CAD build for the part. Positions are in the model's coordinates, mm. A direction names the side the tool comes from. Round coordinates to 2 decimals unless told otherwise and drop trailing zeros. Loops run counter-clockwise (first coordinate to the right, second up) from the corner with the lowest first, then second, coordinate; pieces in that order, holes last. Notation, with made-up numbers: M -33,-7.5 L -11,-7.5 A8 ccw -11,5.5 Z; hole C -0.5,-2.75 d1. An arc over 180 degrees is marked long. Use a Markdown table: item, result. Add a question column.
(1) Band-saw the part on D-D, the plane y = 6.5. Write the cut outline in (x, z).
(2) Wall check: L1, parallel to Y at x = -15.5, z = 18.5; L2, parallel to Z at x = 10, y = -1.5; L3, parallel to Y at x = 0, z = 28. Give the ranges that are in metal, low to high.
(3) Which spindle directions (+Z, -Z, +X, -X, +Y, -Y) get a long thin tool onto all of the face, cutting with end or side? Do faces 4 (the face through (7.1, -12, 11)), 5 (the face through (0, -15, 16.5)), 6 (the face through (-0.508, 10.367, 19.74)). Say none if no direction does.
(4) Flat gauge pins, fed straight in: P1, Ø1, axis at x = -1, y = -14.5, coming from the +Z side; P2, Ø12, axis at y = -13, z = 10.5, coming from the -X side; P3, Ø2, axis at x = -0.5, y = -15, coming from the -Z side; P4, Ø10, axis at x = -11, y = -9.5, coming from the -Z side. Where does each tip first touch, or does it go through?
(5) Two-plate mould, pull along X, no slides. Class faces 1 (the face through (-1.56, 11.9, 9.37)), 2 (the face through (0, 7, 29)), 3 (the face through (13.4, 0.09, 18.61)): released by +X, released by -X, zero draft, split by the parting line, or undercut.
(6) Band-saw the part on C-C, the plane z = 25. Write the cut outline in (x, y).
(7) Band-saw the part on B-B, the plane x = 0. Write the cut outline in (y, z).
(8) Band-saw the part on A-A, the plane y = 0. Write the cut outline in (x, z), and give its area (3 significant figures).
from build123d import *

# Parameters (mm, degrees)
SKETCH1_R           = 12
BOSS_EXTRUDE1_DEPTH = 19
SKETCH2_R           = 3.9
BOSS_EXTRUDE2_DEPTH = 1.5
SKETCH3_R           = 2.1
BOSS_EXTRUDE3_DEPTH = 0.8
SKETCH4_R           = 2.5
BOSS_EXTRUDE4_DEPTH = 8.5
CUT_EXTRUDE2_DEPTH  = 6
SKETCH6_W           = 14.2
SKETCH6_H           = 16.3
BOSS_EXTRUDE5_DEPTH = 13.6
SKETCH7_W           = 7
SKETCH7_H           = 1
BOSS_EXTRUDE6_DEPTH = 2


with BuildPart() as part:
    # Sketch1 → Boss-Extrude1 (new body)
    with BuildSketch(Plane.XY):
        Circle(SKETCH1_R)
    extrude(amount=BOSS_EXTRUDE1_DEPTH)

    # Sketch2 → Boss-Extrude2 (add)
    with BuildSketch(Plane.XY.offset(19)):
        with Locations((0, 6.5)):
            Circle(SKETCH2_R)
    extrude(amount=BOSS_EXTRUDE2_DEPTH)

    # Sketch3 → Boss-Extrude3 (add)
    with BuildSketch(Plane.XY.offset(19)):
        with BuildLine():
            Line((-15.5, 3.5), (15.5, 3.5))
            ThreePointArc((15.5, 3.5), (19, 0), (15.5, -3.5))
            Line((15.5, -3.5), (-15.5, -3.5))
            ThreePointArc((-15.5, -3.5), (-19, 0), (-15.5, 3.5))
        make_face()
        with Locations((-15.5, 0)):
            Circle(SKETCH3_R, mode=Mode.SUBTRACT)
        with Locations((15.5, 0)):
            Circle(SKETCH3_R, mode=Mode.SUBTRACT)
    extrude(amount=-BOSS_EXTRUDE3_DEPTH)

    # Sketch4 → Boss-Extrude4 (add)
    with BuildSketch(Plane.XY.offset(20.5)):
        with Locations((0, 6.5)):
            Circle(SKETCH4_R)
    extrude(amount=BOSS_EXTRUDE4_DEPTH)

    # Sketch5 → Cut-Extrude2 (cut)
    with BuildSketch(Plane.XY.offset(29)):
        with BuildLine():
            Line((-2, 8), (2, 8))
            ThreePointArc((2, 8), (0, 9), (-2, 8))
        make_face()
        with BuildLine():
            Line((2, 5), (-2, 5))
            ThreePointArc((-2, 5), (0, 4), (2, 5))
        make_face()
    extrude(amount=-CUT_EXTRUDE2_DEPTH, mode=Mode.SUBTRACT)

    # Sketch6 → Boss-Extrude5 (add)
    with BuildSketch(Plane(origin=(0, 0, 0), x_dir=(1, 0, 0), z_dir=(0, 1, 0))):
        with Locations((0, -10.85)):
            Rectangle(SKETCH6_W, SKETCH6_H)
    extrude(amount=-BOSS_EXTRUDE5_DEPTH)

    # Sketch7 → Boss-Extrude6 (add)
    with BuildSketch(Plane.XZ.offset(13.6)):
        with Locations((-0.219512042, 17)):
            Rectangle(SKETCH7_W, SKETCH7_H)
    extrude(amount=BOSS_EXTRUDE6_DEPTH)


solid = part.part
Return value:
| question | item | result |
|---|---|---|
| 1 | outline | M -10.09,0 L 10.09,0 L 10.09,19 L 3.9,19 L 3.9,20.5 L 2.5,20.5 L 2.5,29 L -2.5,29 L -2.5,20.5 L -3.9,20.5 L -3.9,19 L -10.09,19 Z |
| 2 | L1 | -3.5 to -2.1, 2.1 to 3.5 |
| 2 | L2 | 0 to 19 |
| 2 | L3 | 5 to 8 |
| 3 | face 4 | +Z, -Z, +X, -Y |
| 3 | face 5 | -Z, +X, -X, -Y |
| 3 | face 6 | +Z |
| 4 | P1 | z = 17.5 |
| 4 | P2 | x = -9.75 |
| 4 | P3 | z = 16.5 |
| 4 | P4 | z = 0 |
| 5 | face 1 | split by the parting line |
| 5 | face 2 | zero draft |
| 5 | face 3 | undercut |
| 6 | outline | M -2,5 L 2,5 A2.5 ccw 2,8 L -2,8 A2.5 ccw Z |
| 7 | outline | M -15.6,16.5 L -13.6,16.5 L -13.6,2.7 L -12,2.7 L -12,0 L 12,0 L 12,19 L 10.4,19 L 10.4,20.5 L 9,20.5 L 9,23 L 8,23 L 8,29 L 5,29 L 5,23 L 4,23 L 4,20.5 L 2.6,20.5 L 2.6,19 L -13.6,19 L -13.6,17.5 L -15.6,17.5 Z |
| 8 | outline | M -19,18.2 L -17.6,18.2 L -17.6,19 L -19,19 Z; M -13.4,18.2 L -12,18.2 L -12,0 L 12,0 L 12,18.2 L 13.4,18.2 L 13.4,19 L -13.4,19 Z; M 17.6,18.2 L 19,18.2 L 19,19 L 17.6,19 Z |
| 8 | area | 460 mm^2 |
